For this review, take the finished solid that the model builds, in its own axes (mm). A direction names the side the tool comes from. Round coordinates to 2 decimals unless told otherwise and drop trailing zeros. Loops run counter-clockwise (first coordinate to the right, second up) from the corner with the lowest first, then second, coordinate; pieces in that order, holes last. Notation, with made-up numbers: (-8, 25.5) -> (47, 25.5) arc R21 ccw to (47, 55.5) -> close; hole circle Ø6 at (39.5, 24). An arc over 180 degrees is marked (long way). Write each question's results on one line, items separated by ' | '.
```python
from build123d import *

# Parameters (mm, degrees)
RESSALTO_EXTRUS_O1_DEPTH          = 10
CORTE_EXTRUS_O1_REACH             = 114.894
ESBO_O4_W                         = 8
ESBO_O4_H                         = 3
CORTE_EXTRUS_O1_DIRECTION_2_REACH = 114.894
FILETE1_R                         = 5
ESBO_O7_R                         = 1.75
CORTE_EXTRUS_O3_DEPTH             = 15
FILETE2_R                         = 5


with BuildPart() as part:
    # Esboço1 → Ressalto-extrusão1 (new, symmetric)
    with BuildSketch(Plane.XY):
        Polygon((0, 0), (4, -3), (4, 2), (24.3, 2), (24.3, -18), (143.3, -18), (143.3, 14), (137.3, 14), (137.3, 0), (32.3, 0), (32.3, 14), (26.3, 14), (26.3, 8), (0, 8), align=None)
        with BuildLine():
            Line((34.3, -10), (54.3, -10))
            ThreePointArc((54.3, -10), (56.3, -12), (54.3, -14))
            Line((54.3, -14), (34.3, -14))
            ThreePointArc((34.3, -14), (32.3, -12), (34.3, -10))
        make_face(mode=Mode.SUBTRACT)
        with BuildLine():
            Line((74.8, -10), (94.8, -10))
            ThreePointArc((94.8, -10), (96.8, -12), (94.8, -14))
            Line((94.8, -14), (74.8, -14))
            ThreePointArc((74.8, -14), (72.8, -12), (74.8, -10))
        make_face(mode=Mode.SUBTRACT)
        with BuildLine():
            Line((115.3, -10), (135.3, -10))
            ThreePointArc((135.3, -10), (137.3, -12), (135.3, -14))
            Line((135.3, -14), (115.3, -14))
            ThreePointArc((115.3, -14), (113.3, -12), (115.3, -10))
        make_face(mode=Mode.SUBTRACT)
    extrude(amount=RESSALTO_EXTRUS_O1_DEPTH, both=True)

    # Esboço2 → Corte-Revolução1 (revolve, cut)
    with BuildSketch(Plane.XY):
        Polygon((27.8, 11), (141.8, 11), (141.8, 7), (137.3, 7), (137.3, -7), (121.3, -7), (104.8, -4), (64.8, -4), (48.3, -7), (32.3, -7), (32.3, 7), (27.8, 7), align=None)
    revolve(axis=Axis((27.8, 11, 0), (1, 0, 0)), mode=Mode.SUBTRACT)

    # Corte-extrusão1: up to this face of the body (flat: up to its plane)
    corte_extrus_o1_end = Plane(part.part.faces().sort_by_distance((27.8, 10.735267855, 0))[0])
    # Esboço4 → Corte-extrusão1 (cut, up to the picked face)
    with BuildSketch(Plane(origin=(32.3, 0, 0), x_dir=(0, 0, -1), z_dir=(1, 0, 0)), mode=Mode.PRIVATE) as corte_extrus_o1_sk1:
        with Locations((0, 12.5)):
            Rectangle(ESBO_O4_W, ESBO_O4_H)
    corte_extrus_o1_tool1 = split(extrude(corte_extrus_o1_sk1.sketch, amount=-CORTE_EXTRUS_O1_REACH, mode=Mode.PRIVATE), bisect_by=corte_extrus_o1_end, keep=Keep.BOTH, mode=Mode.PRIVATE)
    add(corte_extrus_o1_tool1.solids().sort_by(Axis((32.3, 12.5, 0), (-1, 0, 0)))[0], mode=Mode.SUBTRACT)

    # Corte-extrusão1 direction 2: up to this face of the body (flat: up to its plane)
    corte_extrus_o1_direction_2_end = Plane(part.part.faces().sort_by_distance((141.8, 10.735267855, 0))[0])
    # Esboço4 → Corte-extrusão1 direction 2 (cut, up to the picked face)
    with BuildSketch(Plane(origin=(32.3, 0, 0), x_dir=(0, 0, -1), z_dir=(1, 0, 0)), mode=Mode.PRIVATE) as corte_extrus_o1_direction_2_sk1:
        with Locations((0, 12.5)):
            Rectangle(ESBO_O4_W, ESBO_O4_H)
    corte_extrus_o1_direction_2_tool1 = split(extrude(corte_extrus_o1_direction_2_sk1.sketch, amount=CORTE_EXTRUS_O1_DIRECTION_2_REACH, mode=Mode.PRIVATE), bisect_by=corte_extrus_o1_direction_2_end, keep=Keep.BOTH, mode=Mode.PRIVATE)
    add(corte_extrus_o1_direction_2_tool1.solids().sort_by(Axis((32.3, 12.5, 0), (1, 0, 0)))[0], mode=Mode.SUBTRACT)

    # Filete1
    # the kernel refuses this fillet: 5 mm, written as the material it takes off along each edge
    with BuildSketch(Plane(origin=(11.8, -18, -10), x_dir=(0, 0, 1), z_dir=(1, 0, 0))) as filete1_piece_1:
        with BuildLine():
            CenterArc((FILETE1_R, -FILETE1_R), FILETE1_R, 90, 90)
            Line((0, -FILETE1_R), (0, 0))
            Line((0, 0), (FILETE1_R, 0))
        make_face()
    extrude(amount=144, mode=Mode.SUBTRACT)
    with BuildSketch(Plane(origin=(11.8, -18, 10), x_dir=(0, 0, -1), z_dir=(1, 0, 0))) as filete1_piece_2:
        with BuildLine():
            CenterArc((FILETE1_R, FILETE1_R), FILETE1_R, 180, 90)
            Line((0, FILETE1_R), (0, 0))
            Line((0, 0), (FILETE1_R, 0))
        make_face()
    extrude(amount=144, mode=Mode.SUBTRACT)

    # Esboço7 → Corte-extrusão3 (cut)
    with BuildSketch(Plane.XZ.offset(-2)):
        with Locations(Location((14.15, 0, 0), (0, 0, 270))):
            Circle(ESBO_O7_R)
    extrude(amount=-CORTE_EXTRUS_O3_DEPTH, mode=Mode.SUBTRACT)

    # Filete2
    filete2_edges = [part.edges().sort_by_distance(p)[0] for p in [
        (26.3, 8, 0),
    ]]
    fillet(filete2_edges, radius=FILETE2_R)


solid = part.part
```
1. Consider section B-B (z = 0). Give the number of separate pieces and of enclosed holes in the cut face, plus the area to 3 significant figures.
Values found:
separate pieces: 2 | enclosed holes: 3 | area: 1,560 mm2
2. Consider section A-A (x = 46.5). State the section outline as (y, z) points.
Values found:
outline: (-18, -5) arc R5 ccw to (-14, -9.9) -> (-14, 9.9) arc R5 ccw to (-18, 5) -> close; (-10, -10) -> (-3.97, -10) arc R18 cw to (-3.97, 10) -> (-10, 10) -> close
3. Consider section C-C (x = 71). State the section outline as (y, z) points.
Values found:
outline: (-18, -5) arc R5 ccw to (-13, -10) -> (-0.18, -10) arc R15 cw to (-0.18, 10) -> (-13, 10) arc R5 ccw to (-18, 5) -> close
4. Consider section D-D (x = 111.5). State the section outline as (y, z) points, plus the area to 3 significant figures.
Values found:
outline: (-18, -5) arc R5 ccw to (-13, -10) -> (-1.77, -10) arc R16.22 cw to (-1.77, 10) -> (-13, 10) arc R5 ccw to (-18, 5) -> close | area: 267 mm2
5. Tool access review of faces 1 (the face through (4, -1, 0)), 2 (the face through (56.3, -12, 0.1)), 3 (the face through (11, 8, 0)), 4 (the face through (112.934, -5.478, 0.168)): name each direction out of +Z, -Z, +X, -X, +Y, -Y from which nothing blocks a thin tool from reaching the whole face with its end or side.
Values found:
face 1: +Z, -Z, -Y | face 2: +Z, -Z | face 3: +Z, -Z, -X, +Y | face 4: +Y
6. Draft analysis for pull direction X (two halves, no side actions). For faces 5 (the face through (143.3, -2, 0)), 6 (the face through (24.8, 9.43, -0.14)), 7 (the face through (40, -7, 0)), state which applies: released by +X, released by -X, zero draft, split by the parting line, or undercut.
Values found:
face 5: released by +X | face 6: released by -X | face 7: undercut
7. For pin 1 (0.8 mm diameter, centred on y = 13.5, z = 4.5, fed in from -X); pin 2 (1.5 mm diameter, centred on x = 114.5, z = -7, fed in from -Y); pin 3 (6 mm diameter, centred on x = 127.5, z = 2.5, fed in from +Y), all flat-tipped, find the tip position at first contact; note any pin that passes through.
Values found:
pin 1: stops at x = 26.3 | pin 2: stops at y = -17.84 | pin 3: stops at y = -6.14
8. To check wall thickness, follow probe 1 along X at (y, z) = (4.25, 0); probe 2 along Z at (x, y) = (14, 4); probe 3 along X at (y, z) = (2.5, -6). State the ranges of each line that lie inside material, in increasing order.
Values found:
probe 1: x = 0 to 12.4, 15.9 to 32.3, 137.3 to 143.3 | probe 2: z = -10 to -1.74, 1.74 to 10 | probe 3: x = 0 to 32.3, 137.3 to 143.3
